Autodesk Inventor part; units mm, degrees
ref_plane "YZ Plane" through (0, 0, 0) normal (1, 0, 0) x (0, 1, 0)
ref_plane "XZ Plane" through (0, 0, 0) normal (0, 1, 0) x (-1, 0, 0)
ref_plane "XY Plane" through (0, 0, 0) normal (0, 0, 1) x (1, 0, 0)
sketch "Sketch1" plane through (0, 0, 0) normal (0, 0, 1) x (1, 0, 0)
  line L0 (100, 150) -> (0, 150)
  circle A0 centre (50, 207.5) radius 37.5
  line L1 (120, 170) -> (-20, 170)
  line L2 (0, 170) -> (100, 170)
  line L3 (100, 170) -> (100, 265)
  line L4 (100, 265) -> (0, 265)
  line L5 (0, 265) -> (0, 170)
  line L6 (-20, 170) -> (-20, 150)
  line L7 (-20, 150) -> (0, 150)
  line L8 (100, 150) -> (120, 150)
  line L9 (120, 150) -> (120, 170)
  point P0 (0, 0)
  dimension "d0" = 75
  dimension "d1" = 140
  dimension "d2" = 95
extrude "Extrusion1" add sketch "Sketch1" along normal blind 5.5
properties part number "anillo2"
Geometry check sheet. Reference: the model listing, model coordinates, mm. A direction names the side the tool comes from. Give positions to 0.01 mm unless a question says otherwise; leave off trailing zeros. Write each loop counter-clockwise with the first axis right and the second up, starting at its lowest first coordinate (ties: lowest second). Pieces come first, ordered by that corner, then holes. Notation, with made-up numbers: (14, 63) -> (29, 63) arc R10 cw to (29, 77) -> close; hole circle Ø6 at (57, 41.25). An arc over 180 degrees is marked (long way). One line per question, with ' | ' between items.
Item 1: Sectioned sample at C-C, the plane z = 4.1. Record the boundary of the cut face in (x, y), plus the area to 3 significant figures.
Determined:
outline: (-20, 150) -> (120, 150) -> (120, 170) -> (100, 170) -> (100, 265) -> (0, 265) -> (0, 170) -> (-20, 170) -> close; hole circle Ø75 at (50, 207.5) | area: 7,880 mm^2
Item 2: Depth check by flat-ended pin: pin 1 (1.6 mm diameter, centred on x = -14, z = 3, fed in from +Y). Enter the tip coordinate at first touch or a pass-through.
Determined:
pin 1: y = 170
Item 3: Access from +Z, -Z, +X, -X, +Y, -Y to the whole of each face (thin tool, end or side, straight path). Record for faces 4 (the flat face through (33, 170, 0)), 5 (the flat face through (-10, 170, 3)), 6 (the flat face through (110, 170, 3)).
Determined:
face 4: -Z, +X, -X, +Y, -Y | face 5: +Z, -Z, -X, +Y | face 6: +Z, -Z, +X, +Y
Item 4: Sectioned sample at A-A, the plane y = 207.5. Record the boundary of the cut face in (x, z).
Determined:
outline: (0, 0) -> (12.5, 0) -> (12.5, 5.5) -> (0, 5.5) -> close; (87.5, 0) -> (100, 0) -> (100, 5.5) -> (87.5, 5.5) -> close
Item 5: Sectioned sample at D-D, the plane x = -11. Record the boundary of the cut face in (y, z).
Determined:
outline: (150, 0) -> (170, 0) -> (170, 5.5) -> (150, 5.5) -> close
Item 6: Draft check along X on faces 1 (the flat face through (120, 160, 3)), 2 (the cylindrical face through (70.16, 175.88, 2.71)), 3 (the flat face through (-20, 160, 3)). Enter one of: released by +X, released by -X, zero draft, split by the parting line, or undercut.
Determined:
face 1: released by +X | face 2: undercut | face 3: released by -X
Item 7: Scan lines: line 1 along Y through (x, z) = (50, 1.2); line 2 along X through (y, z) = (207.5, 3.7); line 3 along Y through (x, z) = (23, 2.65). Record each from-to range of solid material in increasing order.
Determined:
line 1: 150 to 170, 245 to 265 | line 2: 0 to 12.5, 87.5 to 100 | line 3: 150 to 181.48, 233.52 to 265
Item 8: Sectioned sample at B-B, the plane x = 62. Record the boundary of the cut face in (y, z), plus the area to 3 significant figures.
Determined:
outline: (150, 0) -> (171.97, 0) -> (171.97, 5.5) -> (150, 5.5) -> close; (243.03, 0) -> (265, 0) -> (265, 5.5) -> (243.03, 5.5) -> close | area: 242 mm^2
